CAD build for the part. Positions are in the model's coordinates, mm. A direction names the side the tool comes from. Give positions to 0.01 mm unless a question says otherwise; leave off trailing zeros. Write each loop counter-clockwise with the first axis right and the second up, starting at its lowest first coordinate (ties: lowest second). Pieces come first, ordered by that corner, then holes. Notation, with made-up numbers: (50.25, 41.5) - (95.25, 41.5) arc R23 ccw to (95.25, 74.5) - close; hole circle Ø11 at (9.5, 64.25). An arc over 180 degrees is marked (long way). Answer as a JSON object with one key per item and string values.
from build123d import *

# Parameters (mm, degrees)
SKETCH_2_R          = 1.25
SKETCH_2_R_2        = 1.51
EXTRUDE_1_DEPTH     = 3
SKETCH_4_R          = 1.51
EXTRUDE_2_DEPTH     = 4.5
SKETCH_5_R          = 1.51
EXTRUDE_3_DEPTH     = 4.5
SKETCH_7_W          = 94.013150519
SKETCH_7_H          = 65.926721802
CUT_EXTRUDE_1_DEPTH = 0.5


with BuildPart() as part:
    # 草图2 → 凸台-拉伸1 (new body)
    with BuildSketch(Plane(origin=(0, 0, 0), x_dir=(1, 0, 0), z_dir=(0, 1, 0))):
        with BuildLine():
            Line((21, 5), (16, 5))
            Line((16, 5), (16, 16))
            Line((16, 16), (5, 16))
            Line((5, 16), (5, 21))
            ThreePointArc((5, 21), (0, 26), (-5, 21))
            Line((-5, 21), (-5, 16))
            Line((-5, 16), (-16, 16))
            Line((-16, 16), (-16, 5))
            Line((-16, 5), (-21, 5))
            ThreePointArc((-21, 5), (-26, 0), (-21, -5))
            Line((-21, -5), (-16, -5))
            Line((-16, -5), (-16, -16))
            Line((-16, -16), (-5, -16))
            Line((-5, -16), (-5, -21))
            ThreePointArc((-5, -21), (0, -26), (5, -21))
            Line((5, -21), (5, -16))
            Line((5, -16), (16, -16))
            Line((16, -16), (16, -5))
            Line((16, -5), (21, -5))
            ThreePointArc((21, -5), (26, 0), (21, 5))
        make_face()
        with Locations(Location((-14, 14, 0), (0, 0, 270))):
            Circle(SKETCH_2_R, mode=Mode.SUBTRACT)
        with Locations(Location((14, 14, 0), (0, 0, 270))):
            Circle(SKETCH_2_R, mode=Mode.SUBTRACT)
        with Locations(Location((14, -14, 0), (0, 0, 270))):
            Circle(SKETCH_2_R, mode=Mode.SUBTRACT)
        with Locations(Location((-14, -14, 0), (0, 0, 270))):
            Circle(SKETCH_2_R, mode=Mode.SUBTRACT)
        with Locations(Location((21, 0, 0), (0, 0, 270))):
            Circle(SKETCH_2_R_2, mode=Mode.SUBTRACT)
        with Locations(Location((0, 21, 0), (0, 0, 270))):
            Circle(SKETCH_2_R_2, mode=Mode.SUBTRACT)
        with Locations(Location((0, -21, 0), (0, 0, 270))):
            Circle(SKETCH_2_R_2, mode=Mode.SUBTRACT)
        with Locations(Location((-21, 0, 0), (0, 0, 270))):
            Circle(SKETCH_2_R_2, mode=Mode.SUBTRACT)
        Polygon((-12, 0), (-12, 8), (12, 8), (12, 0), (12, -8), (-12, -8), align=None, mode=Mode.SUBTRACT)
        Polygon((0, -11), (5, -11), (5, -14), (0, -14), (-5, -14), (-5, -11), align=None, mode=Mode.SUBTRACT)
    extrude(amount=EXTRUDE_1_DEPTH)

    # 草图4 → 凸台-拉伸2 (add)
    with BuildSketch(Plane(origin=(0, 3, 0), x_dir=(1, 0, 0), z_dir=(0, 1, 0))):
        with BuildLine():
            Line((-16, -5), (-16, 5))
            Line((-16, 5), (-21, 5))
            ThreePointArc((-21, 5), (-26, 0), (-21, -5))
            Line((-21, -5), (-16, -5))
        make_face()
        with Locations(Location((-21, 0, 0), (0, 0, 270))):
            Circle(SKETCH_4_R, mode=Mode.SUBTRACT)
    extrude(amount=EXTRUDE_2_DEPTH)

    # 草图5 → 凸台-拉伸3 (add)
    # profile 1 of 3: a face of its own
    with BuildSketch(Plane(origin=(0, 3, 0), x_dir=(1, 0, 0), z_dir=(0, 1, 0))):
        with BuildLine():
            Line((-5, 16), (5, 16))
            Line((5, 16), (5, 21))
            ThreePointArc((5, 21), (0, 26), (-5, 21))
            Line((-5, 21), (-5, 16))
        make_face()
        with Locations(Location((0, 21, 0), (0, 0, 270))):
            Circle(SKETCH_5_R, mode=Mode.SUBTRACT)
    # profile 2 of 3: a face of its own
    with BuildSketch(Plane(origin=(0, 3, 0), x_dir=(1, 0, 0), z_dir=(0, 1, 0))):
        with BuildLine():
            Line((16, -5), (16, 5))
            Line((16, 5), (21, 5))
            ThreePointArc((21, 5), (26, 0), (21, -5))
            Line((21, -5), (16, -5))
        make_face()
        with Locations(Location((21, 0, 0), (0, 0, 270))):
            Circle(SKETCH_5_R, mode=Mode.SUBTRACT)
    # profile 3 of 3: a face of its own
    with BuildSketch(Plane(origin=(0, 3, 0), x_dir=(1, 0, 0), z_dir=(0, 1, 0))):
        with BuildLine():
            Line((-5, -16), (5, -16))
            Line((5, -16), (5, -21))
            ThreePointArc((5, -21), (0, -26), (-5, -21))
            Line((-5, -21), (-5, -16))
        make_face()
        with Locations(Location((0, -21, 0), (0, 0, 270))):
            Circle(SKETCH_5_R, mode=Mode.SUBTRACT)
    extrude(amount=EXTRUDE_3_DEPTH)

    # 草图7 → 切除-拉伸1 (cut)
    with BuildSketch(Plane(origin=(0, 7.5, 0), x_dir=(1, 0, 0), z_dir=(0, 1, 0))):
        with Locations((4.289349993, -0.293791095)):
            Rectangle(SKETCH_7_W, SKETCH_7_H)
    extrude(amount=-CUT_EXTRUDE_1_DEPTH, mode=Mode.SUBTRACT)


solid = part.part
(1) Saw through at D-D, the plane x = -14. Give the cut face in (y, z).
Answer key:
{"outline": "(0, -16) - (3, -16) - (3, -15.25) - (0, -15.25) - close; (0, -12.75) - (3, -12.75) - (3, 12.75) - (0, 12.75) - close; (0, 15.25) - (3, 15.25) - (3, 16) - (0, 16) - close"}
(2) Saw through at B-B, the plane x = 0. Give the cut face in (y, z).
Answer key:
{"outline": "(0, -26) - (7, -26) - (7, -22.51) - (0, -22.51) - close; (0, -19.49) - (7, -19.49) - (7, -16) - (3, -16) - (3, -8) - (0, -8) - close; (0, 8) - (3, 8) - (3, 11) - (0, 11) - close; (0, 14) - (3, 14) - (3, 16) - (7, 16) - (7, 19.49) - (0, 19.49) - close; (0, 22.51) - (7, 22.51) - (7, 26) - (0, 26) - close"}
(3) Probe L1, parallel to Z at x = 0, y = 5; L2, parallel to X at y = 2.5, z = -1; L3, parallel to Y at x = 1, z = 10.5. List the from-to ranges inside material, lowest first. Write a range as [from, to].
Answer key:
{"L1": "z = [-26, -22.51], [-19.49, -16], [16, 19.49], [22.51, 26]", "L2": "x = [-25.9, -22.13], [-19.87, -12], [12, 19.87], [22.13, 25.9]", "L3": "y = [0, 3]"}
(4) Flat gauge pins, fed straight in: P1, Ø2.5, axis at x = 0, z = 21, coming from the +Y side; P2, Ø1.5, axis at y = 1, z = -4, coming from the +X side; P3, Ø1.5, axis at x = -4, y = 1.5, coming from the -Z side; P4, Ø3, axis at x = 14, z = 14, coming from the +Y side. Where does each tip first touch, or does it go through?
Answer key:
{"P1": "passes through", "P2": "stops at x = 24.8", "P3": "stops at z = -24.8", "P4": "stops at y = 3"}
(5) Saw through at C-C, the plane z = -14. Give the cut face in (x, y).
Answer key:
{"outline": "(-16, 0) - (-15.25, 0) - (-15.25, 3) - (-16, 3) - close; (-12.75, 0) - (12.75, 0) - (12.75, 3) - (-12.75, 3) - close; (15.25, 0) - (16, 0) - (16, 3) - (15.25, 3) - close"}
(6) 3-axis set-ups, long thin cutter, end or side, ignore diameter. For faces 1 (the face through (0, 1, -8)), 2 (the face through (0, 3, -11)), 3 (the face through (-16, 5, 0)), 4 (the face through (10, 1, 16)): which of +Z, -Z, +X, -X, +Y, -Y reach the whole face in a straight line?
Answer key:
{"face 1": "+Y, -Y", "face 2": "+Y", "face 3": "+Z, -Z, +Y", "face 4": "+Z, +X, +Y, -Y"}
(7) Saw through at A-A, the plane y = 4.25. Give the cut face in (x, z), and give its area (3 significant figures).
Answer key:
{"outline": "(-21, -5) - (-16, -5) - (-16, 5) - (-21, 5) arc R5 ccw to start; (-5, -21) arc R5 ccw to (5, -21) - (5, -16) - (-5, -16) - close; (-5, 16) - (5, 16) - (5, 21) arc R5 ccw to (-5, 21) - close; (16, -5) - (21, -5) arc R5 ccw to (21, 5) - (16, 5) - close; hole circle Ø3.02 at (-21, 0); hole circle Ø3.02 at (0, -21); hole circle Ø3.02 at (0, 21); hole circle Ø3.02 at (21, 0)", "area": "328 mm²"}
(8) Pull direction X, two halves, no side cores. Call faces 5 (the face through (0, 3, -26)), 6 (the face through (-26, 3, 0)), 7 (the face through (1.273, 3.451, -20.188)), 8 (the face through (-19, 3, 5)): pulls with the +X half, pulls with the -X half, needs draft (parallel to the pull), parting line crosses it, or undercut.
Answer key:
{"face 5": "parting line crosses it", "face 6": "pulls with the -X half", "face 7": "undercut", "face 8": "needs draft"}
